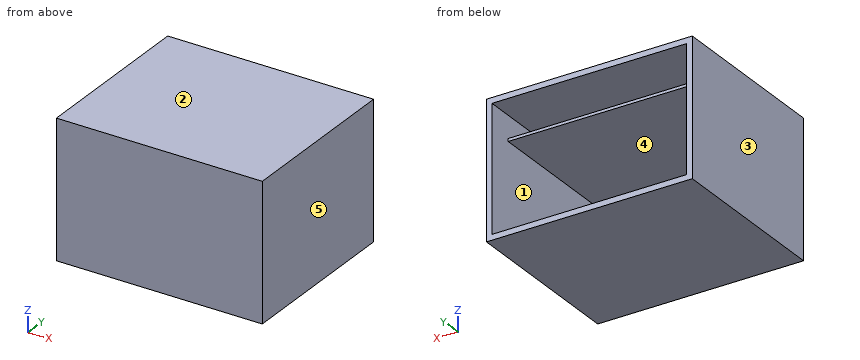
from build123d import *

# Parameters (mm, degrees)
SKETCH1_W           = 370
SKETCH1_H           = 245
BOSS_EXTRUDE1_DEPTH = 10
SKETCH2_W           = 370
SKETCH2_H           = 245
SKETCH2_W_2         = 350
SKETCH2_H_2         = 225
SKETCH2_H_3         = 5
BOSS_EXTRUDE3_DEPTH = 300
SKETCH3_W           = 350
SKETCH3_H           = 5
CUT_EXTRUDE1_DEPTH  = 45


with BuildPart() as part:
    # Sketch1 → Boss-Extrude1 (new body)
    with BuildSketch(Plane(origin=(0, 0, 0), x_dir=(1, 0, 0), z_dir=(0, 1, 0))):
        Rectangle(SKETCH1_W, SKETCH1_H)
    extrude(amount=BOSS_EXTRUDE1_DEPTH)

    # Sketch2 → Boss-Extrude3 (add)
    # profile 1 of 2: a face of its own
    with BuildSketch(Plane(origin=(0, 10, 0), x_dir=(1, 0, 0), z_dir=(0, 1, 0))):
        Rectangle(SKETCH2_W, SKETCH2_H)
        Rectangle(SKETCH2_W_2, SKETCH2_H_2, mode=Mode.SUBTRACT)
    # profile 2 of 2: a face of its own
    with BuildSketch(Plane(origin=(0, 10, 0), x_dir=(1, 0, 0), z_dir=(0, 1, 0))):
        with Locations((0, -70)):
            Rectangle(SKETCH2_W_2, SKETCH2_H_3)
    extrude(amount=BOSS_EXTRUDE3_DEPTH)

    # Sketch3 → Cut-Extrude1 (cut)
    with BuildSketch(Plane(origin=(0, 310, 0), x_dir=(1, 0, 0), z_dir=(0, 1, 0))):
        with Locations((0, -70)):
            Rectangle(SKETCH3_W, SKETCH3_H)
    extrude(amount=-CUT_EXTRUDE1_DEPTH, mode=Mode.SUBTRACT)


solid = part.part
For this review, take the finished solid that the model builds, in its own axes (mm). Face numbers are marked on the shaded views. A direction names the side the tool comes from. Give positions to 0.01 mm unless a question says otherwise; leave off trailing zeros. Loops run counter-clockwise (first coordinate to the right, second up) from the corner with the lowest first, then second, coordinate; pieces in that order, holes last. Notation, with made-up numbers: M 2.5,35.25 L 29.5,35.25 A23 cw 29.5,43.25 Z; hole C -17.75,67.5 d5. An arc over 180 degrees is marked long. Answer as a JSON object with one key per item and string values. Group by question number.
Q1. Insertion check: P1, Ø4, axis at x = -46.5, z = 44, coming from the +Y side; P2, Ø1.5, axis at x = 85, z = 70, coming from the +Y side. Each pin has a flat end and moves straight along its axis. Give the tip position at first contact, or say it passes through.
Q2. Add section A-A on y = 87.5. Give the boundary of the cut face in (x, z), and give its area (4 significant figures).
Q3. Add section D-D on z = -12. Give the boundary of the cut face in (x, y).
Q4. For probe 1 along Z at (x, y) = (-167, 138.5); probe 2 along X at (y, z) = (235.5, -11.5); probe 3 along Z at (x, y) = (-18, 274.5), list the stretches that pass through material, from the lowest coordinate up. Write a range as [from, to].
Q5. Add section B-B on y = 274. Give the boundary of the cut face in (x, z).
Q6. Mouldability with a two-part tool opening along Z and no side actions: class the marked faces 1, 2 and 3 as +Z half, -Z half, draft (parallel to the pull), parting line (faces both ways), or undercut.
Q7. Add section C-C on x = -99.5. Give the boundary of the cut face in (y, z).
Q8. Tool access review of the marked faces 4 and 5: name each direction out of +Z, -Z, +X, -X, +Y, -Y from which nothing blocks a thin tool from reaching the whole face with its end or side.
Checked values:
{
 "1": {"P1": "y = 10", "P2": "y = 265"},
 "2": {"outline": "M -185,-122.5 L 185,-122.5 L 185,122.5 L -185,122.5 Z; hole M -175,-112.5 L 175,-112.5 L 175,67.5 L -175,67.5 Z; hole M -175,72.5 L 175,72.5 L 175,112.5 L -175,112.5 Z", "area": "13,650 mm²"},
 "3": {"outline": "M -185,0 L 185,0 L 185,310 L 175,310 L 175,10 L -175,10 L -175,310 L -185,310 Z"},
 "4": {"probe 1": "[-122.5, -112.5], [67.5, 72.5], [112.5, 122.5]", "probe 2": "[-185, -175], [175, 185]", "probe 3": "[-122.5, -112.5], [112.5, 122.5]"},
 "5": {"outline": "M -185,-122.5 L 185,-122.5 L 185,122.5 L -185,122.5 Z; hole M -175,-112.5 L 175,-112.5 L 175,112.5 L -175,112.5 Z"},
 "6": {"face 1": "undercut", "face 2": "+Z half", "face 3": "draft"},
 "7": {"outline": "M 0,-122.5 L 310,-122.5 L 310,-112.5 L 10,-112.5 L 10,67.5 L 265,67.5 L 265,72.5 L 10,72.5 L 10,112.5 L 310,112.5 L 310,122.5 L 0,122.5 Z"},
 "8": {"face 4": "+Y", "face 5": "+Z, -Z, +X, +Y, -Y"}
}
